```python
from build123d import *

# Parameters (mm, degrees)
PAD_DEPTH      = 50.8
PAD_DEPTH_BACK = 101.6
SKETCH001_R    = 3.175
POCKET_DEPTH   = 1.6002


with BuildPart() as leg1:
    # Sketch → Pad (new body, two sides)
    with BuildSketch(Plane.XY) as pad_sk:
        Polygon((0, 0), (38.1, 0), (38.1, -1.6002), (1.6002, -1.6002), (1.6002, -38.1), (0, -38.1), align=None)
    extrude(amount=PAD_DEPTH)
    extrude(pad_sk.sketch, amount=-PAD_DEPTH_BACK)

    # Sketch001 → Pocket (cut)
    with BuildSketch(Plane(origin=(0, 0, 0), x_dir=(0, -1, 0), z_dir=(-1, 0, 0))):
        with Locations((25.4, -12.7)):
            Circle(SKETCH001_R)
        with Locations((14.3002, -23.7998)):
            Circle(SKETCH001_R)
    extrude(amount=-POCKET_DEPTH, mode=Mode.SUBTRACT)


with BuildPart() as leg1_1:
    # Clone006 placement: moved
    add(leg1.part.moved(Location((-130.837, 130.837, 0))))


with BuildPart() as leg2:
    # Part__Mirroring006: instance of leg1
    add(leg1_1.part.mirror(Plane(origin=(0, 0, 0), x_dir=(1, 0, 0), z_dir=(0, 1, 0))))


with BuildPart() as leg3:
    # Part__Mirroring007: instance of leg2
    add(leg2.part.mirror(Plane(origin=(0, 0, 0), x_dir=(0, -1, 0), z_dir=(1, 0, 0))))


with BuildPart() as leg4:
    # Part__Mirroring008: instance of leg3
    add(leg3.part.mirror(Plane(origin=(0, 0, 0), x_dir=(1, 0, 0), z_dir=(0, 1, 0))))


solid = leg4.part
```
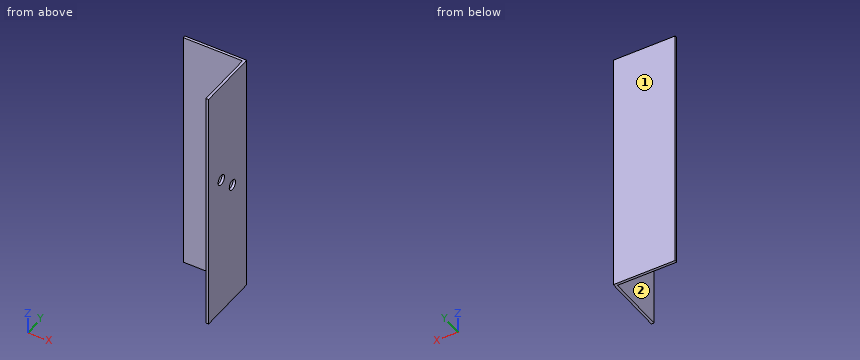
Part model, mm, in its own coordinate system. Face numbers are marked on the shaded views. A direction names the side the tool comes from. Round coordinates to 2 decimals unless told otherwise and drop trailing zeros. Write each loop counter-clockwise with the first axis right and the second up, starting at its lowest first coordinate (ties: lowest second). Pieces come first, ordered by that corner, then holes. Notation, with made-up numbers: (61, 66) -> (95, 66) arc R20 cw to (95, 89) -> close; hole circle Ø7 at (18, 24.5). An arc over 180 degrees is marked (long way). Return JSON: item names as keys, results as strings. Group by question number.
Q1. Pin check, flat tips, straight feed: pin 1 (8.5 mm diameter, centred on y = 116.54, z = -23.8, fed in from -X); pin 2 (18 mm diameter, centred on x = 103, z = -29.5, fed in from -Y); pin 3 (5 mm diameter, centred on y = 105.437, z = -12.7, fed in from +X). Stop position of each tip, or through.
Q2. Saw through at A-A on z = -12.7. Write the cut outline in (x, y), plus the area to 3 significant figures.
Q3. Saw through at C-C on z = -59.5. Write the cut outline in (x, y).
Q4. Which spindle directions (+Z, -Z, +X, -X, +Y, -Y) get a long thin tool onto all of the face, cutting with end or side? Do the marked faces 1 and 2. Say none if no direction does.
Q5. Probe L1, parallel to X at y = 99, z = -5.5; L2, parallel to Z at x = 129.5, y = 104. List the from-to ranges inside material, lowest first. Write a range as [from, to].
Q6. Saw through at B-B on y = 98. Write the cut outline in (x, z).
Answer:
{
 "1": {"pin 1": "x = 129.24", "pin 2": "y = 129.24", "pin 3": "through"},
 "2": {"outline": "(92.74, 129.24) -> (129.24, 129.24) -> (129.24, 108.61) -> (130.84, 108.61) -> (130.84, 130.84) -> (92.74, 130.84) -> close; (129.24, 92.74) -> (130.84, 92.74) -> (130.84, 102.26) -> (129.24, 102.26) -> close", "area": "109 mm2"},
 "3": {"outline": "(92.74, 129.24) -> (129.24, 129.24) -> (129.24, 92.74) -> (130.84, 92.74) -> (130.84, 130.84) -> (92.74, 130.84) -> close"},
 "4": {"face 1": "+Z, -Z, +X, -X, +Y", "face 2": "+Z, -Z, -X, -Y"},
 "5": {"L1": "[129.24, 130.84]", "L2": "[-101.6, -15.53], [-9.87, 50.8]"},
 "6": {"outline": "(129.24, -101.6) -> (130.84, -101.6) -> (130.84, 50.8) -> (129.24, 50.8) -> close"}
}
